CAD build for the part. Positions are in the model's coordinates, mm. A direction names the side the tool comes from. Give positions to 0.01 mm unless a question says otherwise; leave off trailing zeros. Order: outer loops, then holes, each group sorted by start corner. A loop starts at its lowest first (then second) coordinate and runs counter-clockwise, first axis right, second up.
Autodesk Inventor part; units mm, degrees
ref_plane "YZ Plane" through (0, 0, 0) normal (1, 0, 0) x (0, 1, 0)
ref_plane "XZ Plane" through (0, 0, 0) normal (0, 1, 0) x (-1, 0, 0)
ref_plane "XY Plane" through (0, 0, 0) normal (0, 0, 1) x (1, 0, 0)
sketch "Sketch1" plane through (0, 0, 0) normal (0, 1, 0) x (-1, 0, 0)
  circle A0 centre (0, 0) radius 2.921
  dimension "d0" = 5.842
extrude "Extrusion1" add sketch "Sketch1" along normal blind 6.35
sketch "Sketch2" plane through (0, 0, 0) normal (0, -1, 0) x (1, 0, 0)
  circle A0 centre (0, 0) radius 2.921
  line L0 (-4.1275, -0.4128) -> (4.1275, -0.4128)
  line L1 (4.1275, -0.4128) -> (4.1275, 0.4128)
  line L2 (4.1275, 0.4128) -> (-4.1275, 0.4128)
  line L3 (-4.1275, 0.4128) -> (-4.1275, -0.4128)
  line L4 (-4.1275, -0.4128) -> (4.1275, 0.4128) construction
  line L5 (4.1275, -0.4128) -> (-4.1275, 0.4128) construction
  line L6 (3.7809, 1.7063) -> (3.3681, 2.4212)
  line L7 (-3.3681, -2.4212) -> (3.7809, 1.7063)
  line L8 (3.3681, 2.4212) -> (-3.7809, -1.7063)
  line L9 (-3.7809, -1.7063) -> (-3.3681, -2.4212)
  line L10 (2.4212, 3.3681) -> (1.7063, 3.7809)
  line L11 (-1.7063, -3.7809) -> (2.4212, 3.3681)
  line L12 (1.7063, 3.7809) -> (-2.4212, -3.3681)
  line L13 (-2.4212, -3.3681) -> (-1.7063, -3.7809)
  line L14 (0.4128, 4.1275) -> (-0.4127, 4.1275)
  line L15 (0.4127, -4.1275) -> (0.4128, 4.1275)
  line L16 (-0.4127, 4.1275) -> (-0.4128, -4.1275)
  line L17 (-0.4128, -4.1275) -> (0.4127, -4.1275)
  line L18 (-1.7063, 3.7809) -> (-2.4212, 3.3681)
  line L19 (2.4212, -3.3681) -> (-1.7063, 3.7809)
  line L20 (-2.4212, 3.3681) -> (1.7063, -3.7809)
  line L21 (1.7063, -3.7809) -> (2.4212, -3.3681)
  line L22 (-3.3681, 2.4212) -> (-3.7809, 1.7063)
  line L23 (3.7809, -1.7063) -> (-3.3681, 2.4212)
  line L24 (-3.7809, 1.7063) -> (3.3681, -2.4212)
  line L25 (3.3681, -2.4212) -> (3.7809, -1.7063)
  line L26 (-4.1275, 0.4128) -> (-4.1275, -0.4127)
  line L27 (4.1275, 0.4127) -> (-4.1275, 0.4128)
  line L28 (-4.1275, -0.4127) -> (4.1275, -0.4128)
  line L29 (4.1275, -0.4128) -> (4.1275, 0.4127)
  line L30 (-3.7809, -1.7063) -> (-3.3681, -2.4212)
  line L31 (3.3681, 2.4212) -> (-3.7809, -1.7063)
  line L32 (-3.3681, -2.4212) -> (3.7809, 1.7063)
  line L33 (3.7809, 1.7063) -> (3.3681, 2.4212)
  line L34 (-2.4212, -3.3681) -> (-1.7063, -3.7809)
  line L35 (1.7063, 3.7809) -> (-2.4212, -3.3681)
  line L36 (-1.7063, -3.7809) -> (2.4212, 3.3681)
  line L37 (2.4212, 3.3681) -> (1.7063, 3.7809)
  line L38 (-0.4128, -4.1275) -> (0.4127, -4.1275)
  line L39 (-0.4127, 4.1275) -> (-0.4128, -4.1275)
  line L40 (0.4127, -4.1275) -> (0.4128, 4.1275)
  line L41 (0.4128, 4.1275) -> (-0.4127, 4.1275)
  line L42 (1.7063, -3.7809) -> (2.4212, -3.3681)
  line L43 (-2.4212, 3.3681) -> (1.7063, -3.7809)
  line L44 (2.4212, -3.3681) -> (-1.7063, 3.7809)
  line L45 (-1.7063, 3.7809) -> (-2.4212, 3.3681)
  line L46 (3.3681, -2.4212) -> (3.7809, -1.7063)
  line L47 (-3.7809, 1.7063) -> (3.3681, -2.4212)
  line L48 (3.7809, -1.7063) -> (-3.3681, 2.4212)
  line L49 (-3.3681, 2.4212) -> (-3.7809, 1.7063)
  circle A1 centre (0, 0) radius 3.175
  circle A2 centre (0, 0) radius 3.175
  point P0 (2.9327, -1.2166)
  point P1 (3.1481, -0.4127)
  point P2 (3.1481, 0.4128)
  point P3 (2.9327, 1.2166)
  point P4 (2.5199, 1.9315)
  point P5 (1.9315, 2.5199)
  point P6 (1.2166, 2.9327)
  point P7 (0.4128, 3.1481)
  point P8 (-0.4128, 3.1481)
  point P9 (-1.2166, 2.9327)
  point P10 (-1.9315, 2.5199)
  point P11 (-2.5199, 1.9315)
  point P12 (-2.9327, 1.2166)
  point P13 (-3.1481, 0.4127)
  point P14 (-3.1481, -0.4128)
  point P15 (-2.9327, -1.2166)
  point P16 (-2.5199, -1.9315)
  point P17 (-1.9315, -2.5199)
  point P18 (-1.2166, -2.9327)
  point P19 (-0.4128, -3.1481)
  point P20 (0.4127, -3.1481)
  point P21 (1.2166, -2.9327)
  point P22 (1.9315, -2.5199)
  point P23 (2.5199, -1.9315)
  dimension "d5" = 8.255
  dimension "d6" = 0.8255
  dimension "d7" = 360
extrude "Extrusion2" add sketch "Sketch2" along normal blind 3.175
fillet "Fillet1" radius 0.3175 2 edges at (2.4212, -1.5875, 3.3681) (1.7063, -1.5875, 3.7809)
pattern_circular "Circular Pattern1" count 12 over 360 about axis through (0, 0, 0) along (0, 1, 0) of "Fillet1", "Extrusion1"
fillet "Fillet2" radius 0.3175 1 edges at (2.921, 6.35, 0)
sketch "Sketch3" plane through (0, -3.175, 0) normal (0, -1, 0) x (1, 0, 0)
  line L0 (-1.5875, -1.5875) -> (1.5875, -1.5875)
  line L1 (1.5875, -1.5875) -> (1.5875, 1.5875)
  line L2 (1.5875, 1.5875) -> (-1.5875, 1.5875)
  line L3 (-1.5875, 1.5875) -> (-1.5875, -1.5875)
  line L4 (-1.5875, -1.5875) -> (1.5875, 1.5875) construction
  line L5 (1.5875, -1.5875) -> (-1.5875, 1.5875) construction
  point P0 (0, 0)
  dimension "d15" = 3.175
  dimension "d16" = 3.175
extrude "Extrusion3" cut sketch "Sketch3" against normal blind 3.175
properties part number "Gear1"
Item 1: Slice it at A-A (y = 5.75). Give the cut face in (x, z), and give its area (3 significant figures).
Item 2: Wall check: L1, parallel to X at y = -0.5, z = -3.5; L2, parallel to Y at x = -1.75, z = 2.75 (3 decimals); L3, parallel to X at y = 5.75, z = 0. Give the ranges that are in metal, low to high.
Item 3: Tool access for faces 4 (the face through (-0.827, -1.565, 3.065)), 5 (the face through (3.065, -1.565, 0.827)), 6 (the face through (-3.068, -1.565, 0.816)), 7 (the face through (0.633, 2.974, 2.852)), 8 (the face through (0, 0, 0)): list every direction of +Z, -Z, +X, -X, +Y, -Y with a clear straight run to the whole face (end or side of a thin tool).
Item 4: Two-plate mould, pull along Z, no slides. Class faces 1 (the face through (1.588, -2, 0)), 2 (the face through (0.827, -1.565, -3.065)), 3 (the face through (0.816, -1.565, 3.068)): released by +Z, released by -Z, zero draft, split by the parting line, or undercut.
Item 5: Drop flat-ended pins along their axis: pin 1 Ø4 at (y, z) = (0.5, -2.5) entering from +X; pin 2 Ø1 at (x, z) = (0.5, -0.5) entering from -Y; pin 3 Ø0.7 at (y, z) = (-1, -3.5) entering from -X (3 decimals). Give the stop position or say it passes through.
A:
1. outline: circle Ø5.84 at (0, 0)
1. area: 26.8 mm2
2. L1: x = -2.19 to -1.54, -0.41 to 0.41, 1.54 to 2.19
2. L2: y = -3.175 to 0
2. L3: x = -2.92 to 2.92
3. face 4: +Z, +Y, -Y
3. face 5: +X, +Y, -Y
3. face 6: -X, +Y, -Y
3. face 7: +Y
3. face 8: -Y
4. face 1: undercut
4. face 2: released by -Z
4. face 3: released by +Z
5. pin 1: stops at x = 3.66
5. pin 2: stops at y = 0
5. pin 3: stops at x = -2.305
